from build123d import *

# Parameters (mm, degrees)
SKETCH_1_R                    = 30
EXTRUDE_1_DEPTH               = 2
SKETCH_2_R                    = 50
EXTRUDE_2_DEPTH               = 12
EXTRUDE_4_DEPTH               = 45
EXTRUDE_4_DEPTH_BACK          = 32
EXTRUDE_START                 = 12
EXTRUDE_5_DEPTH               = 12
SKETCH_9_R                    = 24
EXTRUDE_6_DEPTH               = 2
CUT_EXTRUDE_1_DEPTH           = 26
SKETCH_11_R                   = 28
CUT_EXTRUDE_2_DEPTH           = 2.5
CUT_EXTRUDE_3_REACH           = 181.761
SKETCH_14_R                   = 12.5
CUT_EXTRUDE_START             = -16
SKETCH_15_R                   = 16
CUT_EXTRUDE_4_DEPTH           = 8
HOLE_WIZARD_M33_1_D           = 29.5
HOLE_WIZARD_M33_1_DEPTH       = 16
HOLE_WIZARD_M33_1_CSINK_D     = 33.05
HOLE_WIZARD_M33_1_CSINK_ANGLE = 90
HOLE_WIZARD_M33_1_TIP         = 8.862694131
CHAMFER_1_SIZE                = 1
FILLET_1_R                    = 1
SKETCH_19_R                   = 24
CUT_EXTRUDE_5_DEPTH           = 2.5
SKETCH_22_R                   = 18
CUT_EXTRUDE_6_DEPTH           = 181.180465165
CHAMFER_2_SIZE                = 1
CUT_EXTRUDE_7_REACH           = 206.494
SKETCH_23_R                   = 6
CUT_EXTRUDE_8_REACH           = 180.264
SKETCH_24_R                   = 6
PATTERN_CIRCULAR_1_COUNT      = 4


# Read off the part's stored shape, not the designer's step: 边界1
with BuildPart() as part:
    # 草图1 → 凸台-拉伸1 (new body)
    with BuildSketch(Plane.XY):
        Circle(SKETCH_1_R)
    extrude(amount=EXTRUDE_1_DEPTH)

    # 草图2 → 凸台-拉伸2 (add)
    with BuildSketch(Plane.XY.offset(2)):
        Circle(SKETCH_2_R)
    extrude(amount=EXTRUDE_2_DEPTH)

    # 草图3 → 旋转1 (revolve)
    with BuildSketch(Plane(origin=(0, 0, 0), x_dir=(1, 0, 0), z_dir=(0, 1, 0))):
        with BuildLine():
            Line((0, -53), (0, -14))
            Line((0, -14), (-22.312803405, -14))
            Line((-22.312803405, -14), (-19, -27.251213621))
            ThreePointArc((-19, -27.251213621), (-28.565713714, -38.577794898), (-32, -53))
            Line((-32, -53), (-32, -135))
            Line((-32, -135), (0, -135))
            Line((0, -135), (0, -53))
        make_face()
    revolve(axis=Axis((0, 0, 135), (0, 0, 1)))

    # 草图5 → 凸台-拉伸4 (add, two sides: drawn at the far end of the back side and taken through both)
    with BuildSketch(Plane(origin=(0, 0, 0), x_dir=(1, 0, 0), z_dir=(0, 1, 0)).offset(-EXTRUDE_4_DEPTH_BACK)):
        with BuildLine():
            Line((-36, -53), (-68, -53))
            Line((-68, -53), (-68, -117))
            Line((-68, -117), (-36, -117))
            ThreePointArc((-36, -117), (-4, -85), (-36, -53))
        make_face()
    extrude(amount=EXTRUDE_4_DEPTH + EXTRUDE_4_DEPTH_BACK)

    # 边界1 outline → 边界1 (revolve)
    with BuildSketch(Plane(origin=(-36, 0, 85), x_dir=(1, 0, 0), z_dir=(0, 0, 1))):
        Polygon((0, -61), (27, -61), (24, -32), (0, -32), align=None)
    revolve(axis=Axis((-36, 0, 85), (0, 1, 0)))

    # 草图8 → 凸台-拉伸5 (add)
    with BuildSketch(Plane(origin=(0, -61, 0), x_dir=(-1, 0, 0), z_dir=(0, -1, 0)).offset(EXTRUDE_START)):
        with BuildLine():
            Line((47.789473684, -55.250910766), (80.631578947, -68.266137306))
            ThreePointArc((80.631578947, -68.266137306), (92, -85), (80.631578947, -101.733862694))
            Line((80.631578947, -101.733862694), (47.789473684, -114.749089234))
            ThreePointArc((47.789473684, -114.749089234), (36, -117), (24.210526316, -114.749089234))
            Line((24.210526316, -114.749089234), (-8.631578947, -101.733862694))
            ThreePointArc((-8.631578947, -101.733862694), (-20, -85), (-8.631578947, -68.266137306))
            Line((-8.631578947, -68.266137306), (24.210526316, -55.250910766))
            ThreePointArc((24.210526316, -55.250910766), (36, -53), (47.789473684, -55.250910766))
        make_face()
    extrude(amount=-EXTRUDE_5_DEPTH)

    # 草图9 → 凸台-拉伸6 (add)
    with BuildSketch(Plane.XZ.offset(73)):
        with Locations(Location((-36, 85, 0), (0, 0, 270))):
            Circle(SKETCH_9_R)
    extrude(amount=EXTRUDE_6_DEPTH)

    # 草图10 → 切除-拉伸1 (cut, symmetric)
    with BuildSketch(Plane.XY.offset(85)):
        with BuildLine():
            Line((0, 26), (-62, 26))
            Line((-62, 26), (-62, -26))
            Line((-62, -26), (0, -26))
            ThreePointArc((0, -26), (26, 0), (0, 26))
        make_face()
    extrude(amount=CUT_EXTRUDE_1_DEPTH, both=True, mode=Mode.SUBTRACT)

    # 草图11 → 切除-拉伸2 (cut)
    with BuildSketch(Plane.XY.offset(135)):
        Circle(SKETCH_11_R)
    extrude(amount=-CUT_EXTRUDE_2_DEPTH, mode=Mode.SUBTRACT)

    # 草图13 → M52x5.0 螺纹孔1 (revolve, cut)
    with BuildSketch(Plane(origin=(0, 0, 132.5), x_dir=(0, -1, 0), z_dir=(1, 0, 0))):
        Polygon((0, 0), (0, 21.5), (23.5, 21.5), (23.5, 2.525), (26.025, 0), align=None)
    revolve(axis=Axis((0, 0, 138.85), (0, 0, -1)), mode=Mode.SUBTRACT)

    # 草图14 → 切除-拉伸3 (cut, up to next)
    with BuildSketch(Plane(origin=(0, 0, 0), x_dir=(-1, 0, 0), z_dir=(0, 0, -1)), mode=Mode.PRIVATE) as cut_extrude_3_sk1:
        Circle(SKETCH_14_R)
    cut_extrude_3_tool1 = extrude(cut_extrude_3_sk1.sketch, amount=-CUT_EXTRUDE_3_REACH, mode=Mode.PRIVATE) & part.part
    add(cut_extrude_3_tool1.solids().sort_by_distance((0, 0, 0))[0], mode=Mode.SUBTRACT)

    # 草图15 → 切除-拉伸4 (cut)
    with BuildSketch(Plane.XY.offset(59).offset(CUT_EXTRUDE_START)):
        Circle(SKETCH_15_R)
    extrude(amount=-CUT_EXTRUDE_4_DEPTH, mode=Mode.SUBTRACT)

    # M33 螺纹孔1
    with Locations(Plane.XY.offset(59)):
        with Locations((0, 0)):
            CounterSinkHole(HOLE_WIZARD_M33_1_D / 2, HOLE_WIZARD_M33_1_CSINK_D / 2, depth=HOLE_WIZARD_M33_1_DEPTH, counter_sink_angle=HOLE_WIZARD_M33_1_CSINK_ANGLE)
            with Locations((0, 0, -(HOLE_WIZARD_M33_1_DEPTH + HOLE_WIZARD_M33_1_TIP / 2))):  # 118° drill point
                Cone(0, HOLE_WIZARD_M33_1_D / 2, HOLE_WIZARD_M33_1_TIP, mode=Mode.SUBTRACT)

    # 倒角1
    chamfer_1_edges = [part.edges().sort_by_distance(p)[0] for p in [
        (14.75, 0, 43),
    ]]
    chamfer(chamfer_1_edges, length=CHAMFER_1_SIZE)

    # 圆角1
    # the kernel refuses this fillet: 1 mm, written as the material it adds along each edge
    with BuildSketch(Plane(origin=(0, 0, 43), x_dir=(1, 0, 0), z_dir=(0, -1, 0))) as fillet_1_piece_1:
        with BuildLine():
            CenterArc((15, -0.661437828), FILLET_1_R, 0, 41.409622109)
            Line((16, -0.661437828), (16.02, -0.661437828))
            Line((16.02, -0.661437828), (16.02, 0))
            Line((16.02, 0), (16, 0.02))
            ThreePointArc((16, 0.02), (15.875, 0.02), (15.765, 0.013228757))
            Line((15.765, 0.013228757), (15.75, 0))
        make_face()
    revolve(axis=Axis((0, 0, 43), (0, 0, 1)))
    with BuildSketch(Plane(origin=(0, 0, 35), x_dir=(1, 0, 0), z_dir=(0, -1, 0))) as fillet_1_piece_2:
        with BuildLine():
            CenterArc((16 - FILLET_1_R, FILLET_1_R), FILLET_1_R, 270, 90)
            Line((16 - FILLET_1_R, 0), (16 - FILLET_1_R, -FILLET_1_R * 0.02))
            Line((16 - FILLET_1_R, -FILLET_1_R * 0.02), (16 + FILLET_1_R * 0.02, -FILLET_1_R * 0.02))
            Line((16 + FILLET_1_R * 0.02, -FILLET_1_R * 0.02), (16 + FILLET_1_R * 0.02, FILLET_1_R))
            Line((16 + FILLET_1_R * 0.02, FILLET_1_R), (16, FILLET_1_R))
        make_face()
    revolve(axis=Axis((0, 0, 35), (0, 0, 1)))

    # 草图19 → 切除-拉伸5 (cut)
    with BuildSketch(Plane(origin=(0, 45, 0), x_dir=(1, 0, 0), z_dir=(0, 1, 0))):
        with Locations(Location((-36, -85, 0), (0, 0, 90))):
            Circle(SKETCH_19_R)
    extrude(amount=-CUT_EXTRUDE_5_DEPTH, mode=Mode.SUBTRACT)

    # 草图21 → M39 螺纹孔1 (revolve, cut)
    with BuildSketch(Plane(origin=(-36, 42.5, 85), x_dir=(0, 0, 1), z_dir=(1, 0, 0))):
        Polygon((0, 0), (0, 16.5), (17.5, 16.5), (17.5, 2.025), (19.525, 0), align=None)
    revolve(axis=Axis((-36, 48.85, 85), (0, -1, 0)), mode=Mode.SUBTRACT)

    # 草图22 → 切除-拉伸6 (cut, through all)
    with BuildSketch(Plane(origin=(0, -26, 0), x_dir=(1, 0, 0), z_dir=(0, 1, 0))):
        with Locations(Location((-36, -85, 0), (0, 0, 270))):
            Circle(SKETCH_22_R)
    extrude(amount=-CUT_EXTRUDE_6_DEPTH, mode=Mode.SUBTRACT)

    # 倒角2
    chamfer_2_edges = [part.edges().sort_by_distance(p)[0] for p in [
        (-36, -75, 67),
    ]]
    chamfer(chamfer_2_edges, length=CHAMFER_2_SIZE)

    # 草图23 → 切除-拉伸7 (cut, up to next)
    with BuildSketch(Plane.XZ.offset(73), mode=Mode.PRIVATE) as cut_extrude_7_sk1:
        with Locations(Location((-74, 85, 0), (0, 0, 270))):
            Circle(SKETCH_23_R)
    cut_extrude_7_tool1 = extrude(cut_extrude_7_sk1.sketch, amount=-CUT_EXTRUDE_7_REACH, mode=Mode.PRIVATE) & part.part
    # 草图23 → 切除-拉伸7 (cut, up to next)
    with BuildSketch(Plane.XZ.offset(73), mode=Mode.PRIVATE) as cut_extrude_7_sk2:
        with Locations(Location((2, 85, 0), (0, 0, 270))):
            Circle(SKETCH_23_R)
    cut_extrude_7_tool2 = extrude(cut_extrude_7_sk2.sketch, amount=-CUT_EXTRUDE_7_REACH, mode=Mode.PRIVATE) & part.part
    add(cut_extrude_7_tool1.solids().sort_by_distance((-74, -73, 85))[0], mode=Mode.SUBTRACT)
    add(cut_extrude_7_tool2.solids().sort_by_distance((2, -73, 85))[0], mode=Mode.SUBTRACT)

    # 草图24 → 切除-拉伸8 (cut, up to next)
    with BuildSketch(Plane(origin=(0, 0, 2), x_dir=(-1, 0, 0), z_dir=(0, 0, -1)), mode=Mode.PRIVATE) as cut_extrude_8_sk1:
        with Locations((28.284271247, 28.284271247)):
            Circle(SKETCH_24_R)
    cut_extrude_8_tool1 = extrude(cut_extrude_8_sk1.sketch, amount=-CUT_EXTRUDE_8_REACH, mode=Mode.PRIVATE) & part.part
    cut_extrude_8 = cut_extrude_8_tool1.solids().sort_by_distance((-28.284271, 28.284271, 2))[0]
    add(cut_extrude_8, mode=Mode.SUBTRACT)

    # 阵列(圆周)1: 切除-拉伸8 ×4 about axis
    pattern_circular_1_axis = Axis((0, 0, 0), (0, 0, 1))
    for i in range(1, PATTERN_CIRCULAR_1_COUNT):
        add(cut_extrude_8.rotate(pattern_circular_1_axis, i * 360 / PATTERN_CIRCULAR_1_COUNT), mode=Mode.SUBTRACT)


solid = part.part
Design review of the part built by this model. Coordinates are the model's own, in mm. A direction names the side the tool comes from. Round coordinates to 2 decimals unless told otherwise and drop trailing zeros. Order: outer loops, then holes, each group sorted by start corner. A loop starts at its lowest first (then second) coordinate and runs counter-clockwise, first axis right, second up.
1) Consider section A-A (x = -74). State the section outline as (y, z) points.
The answers:
outline: (-73, 65.64) - (-61, 65.64) - (-61, 79) - (-73, 79) - close; (-73, 91) - (-61, 91) - (-61, 104.36) - (-73, 104.36) - close
2) Machinability: for faces 1 (the cylindrical face through (-50.6, -73.99, 104.05)), 2 (the flat face through (-52, 6, 117)), 3 (the cylindrical face through (-36, -67, 117)), 4 (the conical face through (2.54, -19.36, 25.14)), which of the approach directions +Z, -Z, +X, -X, +Y, -Y give a long, thin tool a straight path to every point of the face, cutting with its end or side? Answer none if there is none.
The answers:
face 1: -Y
face 2: +Z, -X, +Y, -Y
face 3: +Z, -Y
face 4: none
3) Consider section C-C (z = 121). State the section outline as (x, y) points.
The answers:
outline: circle Ø64 at (0, 0); hole circle Ø47 at (0, 0)
4) Consider section B-B (y = -63). State the section outline as (x, z) points, plus the area to 3 significant figures.
The answers:
outline: (-80.63, 68.27) - (-47.79, 55.25) arc R32 ccw to (-24.21, 55.25) - (8.63, 68.27) arc R18 ccw to (8.63, 101.73) - (-24.21, 114.75) arc R32 ccw to (-47.79, 114.75) - (-80.63, 101.73) arc R18 ccw to start; hole circle Ø12 at (-74, 85); hole circle Ø36 at (-36, 85); hole circle Ø12 at (2, 85)
area: 3,830 mm2
5) Consider section D-D (x = 2). Count the separate pieces of the cut face and the enclosed holes in it, plus the area to 3 significant figures.
The answers:
separate pieces: 4
enclosed holes: 0
area: 3,430 mm2
6) Draft analysis for pull direction Z (two halves, no side actions). For faces 5 (the flat face through (-24, -73, 63)), 6 (the flat face through (-7.56, -67.08, 61.85)), 7 (the flat face through (-17.7, -26, 85.4)), state which applies: released by +Z, released by -Z, zero draft, split by the parting line, or undercut.
The answers:
face 5: zero draft
face 6: released by -Z
face 7: undercut
7) For L1, parallel to X at y = -68.5, z = 85; L2, parallel to Y at x = 0, z = 8; L3, parallel to Y at x = 0, z = 134, list the stretches that pass through material, from the lowest coordinate up.
The answers:
L1: x = -92 to -80, -68 to -54, -18 to -4, 8 to 20
L2: y = -50 to -12.5, 12.5 to 50
L3: y = -32 to -28, 28 to 32
8) Clearance check with flat-ended pins moving along their axes: pin 1 Ø15.5 at (x, z) = (-43, 81) entering from +Y; pin 2 Ø9.5 at (x, y) = (-28.28, 28.28) entering from -Z; pin 3 Ø19 at (x, z) = (-18, 77) entering from +Y; pin 4 Ø1.5 at (x, y) = (1.5, -50.5) entering from +Z. State where each tip first meets the part, or that it passes through.
The answers:
pin 1: passes through
pin 2: stops at z = 53.14
pin 3: stops at y = 45
pin 4: stops at z = 14
